Here's how the part is built. I have some questions about the finished solid (model axes, mm). Coordinates: 2 decimals unless noted, no trailing zeros. Loops run counter-clockwise (first coordinate to the right, second up) from the corner with the lowest first, then second, coordinate; pieces in that order, holes last. Notation, with made-up numbers: M 34,12 L 82,12 A8 cw 82,20 Z; hole C 82,-13.5 d9. An arc over 180 degrees is marked long. Use one line per item in the form item = value. Start each with the question number.
(1) Will these pins go through, and if not, where does the flat tip stop? P1, Ø1, axis at x = 47.5, y = 0.5, coming from the +Z side; P2, Ø0.6, axis at x = 47, y = 1.5, coming from the -Z side.
(2) Please list where these lines run through material, in increasing order: L1, parallel to X at y = 0.4, z = 28; L2, parallel to Z at x = 45, y = 0.8.
(3) Imagine slicing it at C-C, the plane z = 28. Please give me the cut outline in (x, y).
(4) Imagine slicing it at A-A, the plane y = 1.3. Please give me the cut outline in (x, z).
(5) Thinking about a two-plate mould opening in Z: for faces 1 (the flat face through (-1, 0, -1)), 2 (the cylindrical face through (-28.51, 0.28, -26.38)), which applies, +Z half, -Z half, draft (parallel to the pull), parting line (faces both ways), or undercut?
(6) Imagine slicing it at B-B, the plane x = -28. Please give me the cut outline in (y, z).
```python
from build123d import *

# Parameters (mm, degrees)
SKETCH1_W                                      = 100
SKETCH1_H                                      = 100
BASE_EXTRUSION_DEPTH                           = 2
SKETCH2_W                                      = 9
SKETCH2_H                                      = 9
CORNER_CUTOUTS_DEPTH                           = 71.738956735
CSK_FOR_M3_FLAT_HEAD_MACHINE_SCREW2_AT_2_COUNT = 2
CSK_FOR_M3_FLAT_HEAD_MACHINE_SCREW2_AT_2_PITCH = 56
CSK_FOR_M3_FLAT_HEAD_MACHINE_SCREW2_AT_3_COUNT = 2
CSK_FOR_M3_FLAT_HEAD_MACHINE_SCREW2_AT_3_PITCH = 79.195959493
CSK_FOR_M3_FLAT_HEAD_MACHINE_SCREW2_AT_4_COUNT = 2
CSK_FOR_M3_FLAT_HEAD_MACHINE_SCREW2_AT_4_PITCH = 56
FILLET_FOR_RAILS_R                             = 1


with BuildPart() as part:
    # Sketch1 → Base Extrusion (new body)
    with BuildSketch(Plane(origin=(0, 0, 0), x_dir=(1, 0, 0), z_dir=(0, 1, 0))):
        Rectangle(SKETCH1_W, SKETCH1_H)
    extrude(amount=BASE_EXTRUSION_DEPTH)

    # Sketch2 → Corner Cutouts (cut, through all)
    with BuildSketch(Plane(origin=(0, 2, 0), x_dir=(1, 0, 0), z_dir=(0, 1, 0))):
        with Locations((45.5, 45.5)):
            Rectangle(SKETCH2_W, SKETCH2_H)
        with Locations((-45.5, 45.5)):
            Rectangle(SKETCH2_W, SKETCH2_H)
        with Locations((-45.5, -45.5)):
            Rectangle(SKETCH2_W, SKETCH2_H)
        with Locations((45.5, -45.5)):
            Rectangle(SKETCH2_W, SKETCH2_H)
    extrude(amount=-CORNER_CUTOUTS_DEPTH, mode=Mode.SUBTRACT)

    # Sketch10 → CSK for M3 Flat Head Machine Screw2 (revolve, cut)
    with BuildSketch(Plane(origin=(-28, 2, 28), x_dir=(0, 0, 1), z_dir=(1, 0, 0))):
        Polygon((0, 0), (0, 2), (1.7, 2), (1.7, 1.45), (3.15, 0), align=None)
    csk_for_m3_flat_head_machine_screw2 = revolve(axis=Axis((-28, 8.35, 28), (0, -1, 0)), mode=Mode.SUBTRACT)

    # CSK for M3 Flat Head Machine Screw2 at 2: CSK for M3 Flat Head Machine Screw2 ×2
    with Locations(*[(0, 0, -i * CSK_FOR_M3_FLAT_HEAD_MACHINE_SCREW2_AT_2_PITCH) for i in range(1, CSK_FOR_M3_FLAT_HEAD_MACHINE_SCREW2_AT_2_COUNT)]):
        add(csk_for_m3_flat_head_machine_screw2, mode=Mode.SUBTRACT)

    # CSK for M3 Flat Head Machine Screw2 at 3: CSK for M3 Flat Head Machine Screw2 ×2
    with Locations(*[Vector(0.7071067811865476, 0, -0.7071067811865476) * (i * CSK_FOR_M3_FLAT_HEAD_MACHINE_SCREW2_AT_3_PITCH) for i in range(1, CSK_FOR_M3_FLAT_HEAD_MACHINE_SCREW2_AT_3_COUNT)]):
        add(csk_for_m3_flat_head_machine_screw2, mode=Mode.SUBTRACT)

    # CSK for M3 Flat Head Machine Screw2 at 4: CSK for M3 Flat Head Machine Screw2 ×2
    with Locations(*[(i * CSK_FOR_M3_FLAT_HEAD_MACHINE_SCREW2_AT_4_PITCH, 0, 0) for i in range(1, CSK_FOR_M3_FLAT_HEAD_MACHINE_SCREW2_AT_4_COUNT)]):
        add(csk_for_m3_flat_head_machine_screw2, mode=Mode.SUBTRACT)

    # Fillet For Rails
    fillet_for_rails_edges = [part.edges().sort_by_distance(p)[0] for p in [
        (41, 1, -41),
        (-41, 1, -41),
        (-41, 1, 41),
        (41, 1, 41),
    ]]
    fillet(fillet_for_rails_edges, radius=FILLET_FOR_RAILS_R)


solid = part.part
```
Answer:
q1.P1 = 41
q1.P2 = -41
q2.L1 = -50 to -29.7, -26.3 to 26.3, 29.7 to 50
q2.L2 = -41 to 41
q3.outline = M -50,0 L -29.7,0 L -29.7,0.55 L -31.15,2 L -50,2 Z; M -26.3,0 L 26.3,0 L 26.3,0.55 L 24.85,2 L -24.85,2 L -26.3,0.55 Z; M 29.7,0 L 50,0 L 50,2 L 31.15,2 L 29.7,0.55 Z
q4.outline = M -50,-41 L -42,-41 A1 cw -41,-42 L -41,-50 L 41,-50 L 41,-42 A1 cw 42,-41 L 50,-41 L 50,41 L 42,41 A1 cw 41,42 L 41,50 L -41,50 L -41,42 A1 cw -42,41 L -50,41 Z; hole C -28,-28 d4.9; hole C -28,28 d4.9; hole C 28,-28 d4.9; hole C 28,28 d4.9
q5.face_1 = draft
q5.face_2 = undercut
q6.outline = M 0,-50 L 2,-50 L 2,-31.15 L 0.55,-29.7 L 0,-29.7 Z; M 0,-26.3 L 0.55,-26.3 L 2,-24.85 L 2,24.85 L 0.55,26.3 L 0,26.3 Z; M 0,29.7 L 0.55,29.7 L 2,31.15 L 2,50 L 0,50 Z
